Geometry: final body of the model. Coordinates: model frame, mm. A direction names the side the tool comes from. Give positions to 0.01 mm unless a question says otherwise; leave off trailing zeros. Loops run counter-clockwise (first coordinate to the right, second up) from the corner with the lowest first, then second, coordinate; pieces in that order, holes last. Notation, with made-up numbers: (-12.75, -8.75) -> (46.25, -8.75) arc R27 cw to (46.25, 14.25) -> close; hole circle Ø8 at (39, -26.5). An arc over 180 degrees is marked (long way). Answer in a Markdown table with one row per item. Add a question column.
1) Access query for faces 1 (the flat face through (156.716, 204, 1)), 2 (the flat face through (155, 198.994, 1)). Directions: +Z, -Z, +X, -X, +Y, -Y. A direction counts if a zero-diameter tool reaches every point of the face in a straight line with its end or side. Return the directions, or none.
2) First-contact query: P1, Ø1.5, axis at x = 154.5, y = 202, coming from the +Z side; P2, Ø1.5, axis at x = 153.5, z = 0.5, coming from the +Y side. Flat tips, straight axial feed; report the tip coordinate or a pass-through.
3) Section query B-B (z = 1). Return the cut outline in (x, y).
4) Line query: line 1 (X direction, y = 206, z = 0.45); line 2 (Y direction, x = 155.5, z = 0.4); line 3 (Y direction, x = 155.75, z = 1.1). Output: solid intervals per line, ascending. Write a range as from..to.
5) Section query D-D (y = 212). Return the cut outline in (x, z), plus the area to 3 significant figures.
6) Section query A-A (y = 201.25). Return the cut outline in (x, z), plus the area to 4 significant figures.
7) Draft query along Y for faces 3 (the flat face through (155, 208, 0)), 4 (the cylindrical face through (154.992, 216.993, 1.479)), 5 (the flat face through (155, 206.744, 1)), 6 (the flat face through (153.466, 203, 1)). Return one class per face: +Y half, -Y half, draft (parallel to the pull), parting line (faces both ways), or undercut.
8) Section query C-C (x = 154.5). Return the cut outline in (y, z), plus the area to 3 significant figures.
```python
from build123d import *

# Parameters (mm, degrees)
MODEL_R                 = 1.5
SALIENTE_EXTRUIR1_DEPTH = 3


with BuildPart() as part:
    # Model → Saliente-Extruir1 (new body)
    with BuildSketch(Plane.XY):
        with BuildLine():
            Line((159.591356547, 212.494036843), (159.591356547, 198.994036843))
            Line((159.591356547, 198.994036843), (150.591356547, 198.994036843))
            Line((150.591356547, 198.994036843), (150.591356547, 212.494036843))
            ThreePointArc((150.591356547, 212.494036843), (155.091356547, 216.994036843), (159.591356547, 212.494036843))
        make_face()
        with Locations((155.091356547, 212.494036843)):
            Circle(MODEL_R, mode=Mode.SUBTRACT)
        with BuildLine():
            Line((153.466356547, 200.994036843), (153.466356547, 205.994036843))
            ThreePointArc((153.466356547, 205.994036843), (153.686026462, 206.524366929), (154.216356547, 206.744036843))
            Line((154.216356547, 206.744036843), (155.966356547, 206.744036843))
            ThreePointArc((155.966356547, 206.744036843), (156.496686633, 206.524366929), (156.716356547, 205.994036843))
            Line((156.716356547, 205.994036843), (156.716356547, 200.994036843))
            ThreePointArc((156.716356547, 200.994036843), (156.496686633, 200.463706757), (155.966356547, 200.244036843))
            Line((155.966356547, 200.244036843), (154.216356547, 200.244036843))
            ThreePointArc((154.216356547, 200.244036843), (153.686026462, 200.463706757), (153.466356547, 200.994036843))
        make_face(mode=Mode.SUBTRACT)
    extrude(amount=SALIENTE_EXTRUIR1_DEPTH)


solid = part.part
```
Evaluation:
| question | item | result |
|---|---|---|
| 1 | face 1 | +Z, -Z |
| 1 | face 2 | +Z, -Z, +X, -X, -Y |
| 2 | P1 | through |
| 2 | P2 | y = 216.91 |
| 3 | outline | (150.59, 198.99) -> (159.59, 198.99) -> (159.59, 212.49) arc R4.5 ccw to (150.59, 212.49) -> close; hole (153.47, 200.99) arc R0.75 ccw to (154.22, 200.24) -> (155.97, 200.24) arc R0.75 ccw to (156.72, 200.99) -> (156.72, 205.99) arc R0.75 ccw to (155.97, 206.74) -> (154.22, 206.74) arc R0.75 ccw to (153.47, 205.99) -> close; hole circle Ø3 at (155.09, 212.49) |
| 4 | line 1 | 150.59..153.47, 156.72..159.59 |
| 4 | line 2 | 198.99..200.24, 206.74..211.05, 213.94..216.98 |
| 4 | line 3 | 198.99..200.24, 206.74..211.15, 213.84..216.95 |
| 5 | outline | (150.59, 0) -> (153.68, 0) -> (153.68, 3) -> (150.59, 3) -> close; (156.51, 0) -> (159.59, 0) -> (159.59, 3) -> (156.51, 3) -> close |
| 5 | area | 18.5 mm² |
| 6 | outline | (150.59, 0) -> (153.47, 0) -> (153.47, 3) -> (150.59, 3) -> close; (156.72, 0) -> (159.59, 0) -> (159.59, 3) -> (156.72, 3) -> close |
| 6 | area | 17.25 mm² |
| 7 | face 3 | draft |
| 7 | face 4 | +Y half |
| 7 | face 5 | undercut |
| 7 | face 6 | undercut |
| 8 | outline | (198.99, 0) -> (200.24, 0) -> (200.24, 3) -> (198.99, 3) -> close; (206.74, 0) -> (211.12, 0) -> (211.12, 3) -> (206.74, 3) -> close; (213.87, 0) -> (216.96, 0) -> (216.96, 3) -> (213.87, 3) -> close |
| 8 | area | 26.1 mm² |
